The figure shows three views and two pictorial views of one solid part (mm, origin at its lowest corner). Answer the questions. A direction names the side the tool comes from. Give positions to 0.01 mm unless a question says otherwise; leave off trailing zeros. Order: outer loops, then holes, each group sorted by start corner. A loop starts at its lowest first (then second) coordinate and runs counter-clockwise, first axis right, second up. Notation, with made-up numbers: (-37, 31) -> (-7, 31) arc R23 cw to (-7, 42) -> close; hole circle Ø5 at (87, 10). An arc over 180 degrees is marked (long way). Use one line per item in the form item = value.
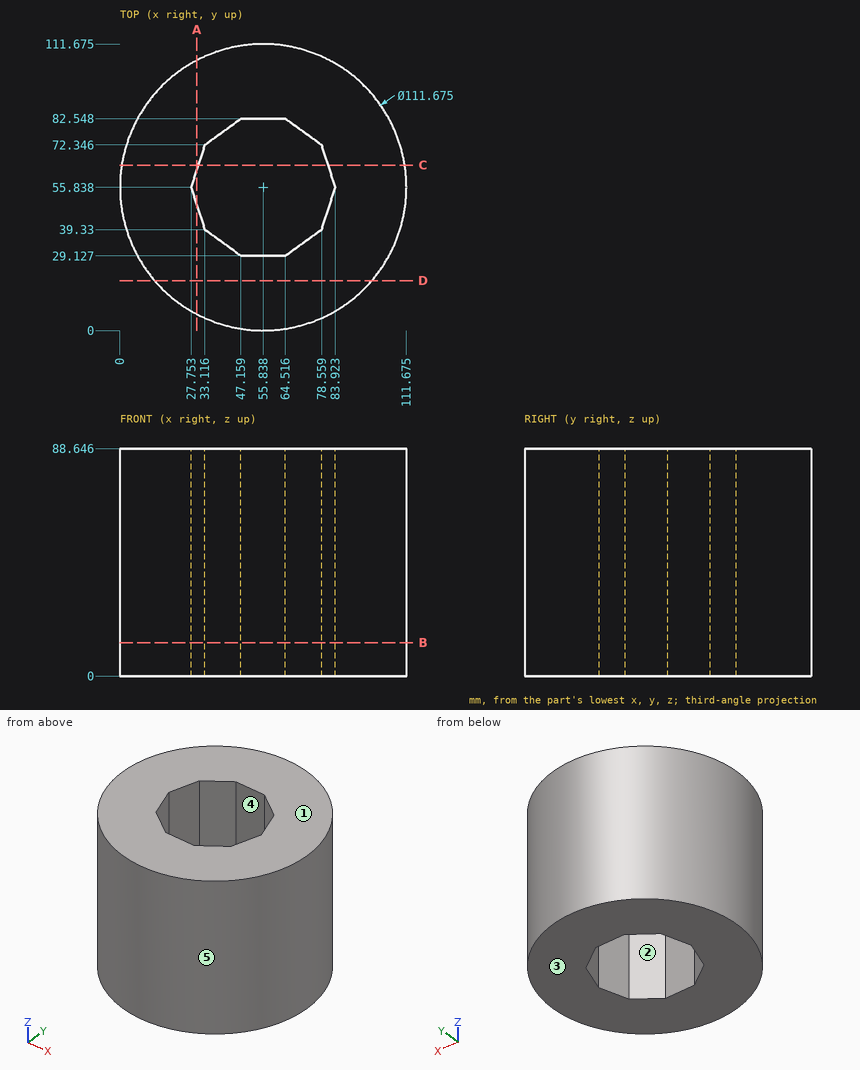
Item 1: Straight lines are drawn through the part: L1, parallel to X at y = 30.5, z = 67 (1 decimal); L2, parallel to Y at x = 41, z = 77 (1 decimal); L3, parallel to Y at x = 35, z = 82 (1 decimal). For each, find the intervals that lie inside material, in ascending order. Write a range as from..to.
Checks:
L1 = 6.1..45.3, 66.4..105.6
L2 = 2..33.6, 78.1..109.7
L3 = 4..38, 73.7..107.6
Item 2: Which of the six approach directions +Z, -Z, +X, -X, +Y, -Y give full straight-line access (tool end or side, diameter ignored) to the marked faces 1 and 2?
Checks:
face_1 = +Z, +X, -X, +Y, -Y
face_2 = +Z, -Z
Item 3: The part is cut by section C-C on y = 64.5. Give the vertices of the cut face in (x, z).
Checks:
outline = (0.68, 0) -> (30.57, 0) -> (30.57, 88.65) -> (0.68, 88.65) -> close; (81.11, 0) -> (111, 0) -> (111, 88.65) -> (81.11, 88.65) -> close
Item 4: The part is cut by section A-A on x = 30. Give the vertices of the cut face in (y, z) (1 decimal), and give its area (3 significant figures).
Checks:
outline = (6.3, 0) -> (48.9, 0) -> (48.9, 88.6) -> (6.3, 88.6) -> close; (62.8, 0) -> (105.3, 0) -> (105.3, 88.6) -> (62.8, 88.6) -> close
area = 7,550 mm²
Item 5: Given pin 1 Ø8 at (x, z) = (20.5, 57) entering from +Y; pin 2 Ø2 at (y, z) = (34, 62.5) entering from +X; pin 3 Ø1.5 at (x, z) = (76.5, 62) entering from -Y, each flat-ended and moving along its own axis, determine where each tip first touches the part or whether it passes through.
Checks:
pin_1 = 102.05
pin_2 = 107.64
pin_3 = 3.67
Item 6: The part is cut by section B-B on z = 13. Give the vertices of the cut face in (x, y) (1 decimal), and give its area (3 significant figures).
Checks:
outline = circle Ø111.7 at (55.8, 55.8); hole (27.8, 55.8) -> (33.1, 39.3) -> (47.2, 29.1) -> (64.5, 29.1) -> (78.6, 39.3) -> (83.9, 55.8) -> (78.6, 72.3) -> (64.5, 82.5) -> (47.2, 82.5) -> (33.1, 72.3) -> close
area = 7,480 mm²
Item 7: Determine the mould class of the marked faces 3, 4 and 5 for opening direction Y: +Y half, -Y half, draft (parallel to the pull), parting line (faces both ways), or undercut.
Checks:
face_3 = draft
face_4 = undercut
face_5 = parting line
Item 8: The part is cut by section D-D on y = 19.5. Give the vertices of the cut face in (x, z).
Checks:
outline = (13.44, 0) -> (98.23, 0) -> (98.23, 88.65) -> (13.44, 88.65) -> close
